from build123d import *

# Parameters (mm, degrees)
SKETCH1_R           = 4.78
BOSS_EXTRUDE1_DEPTH = 2.78
SKETCH2_W           = 6
SKETCH2_H           = 6
BOSS_EXTRUDE2_DEPTH = 10


with BuildPart() as part:
    # Sketch1 → Boss-Extrude1 (new, symmetric)
    with BuildSketch(Plane(origin=(0, 0, 0), x_dir=(0, 0, -1), z_dir=(1, 0, 0))):
        Circle(SKETCH1_R)
    extrude(amount=BOSS_EXTRUDE1_DEPTH, both=True)

    # Sketch2 → Boss-Extrude2 (add)
    with BuildSketch(Plane(origin=(2.78, 0, 0), x_dir=(0, 0, -1), z_dir=(1, 0, 0))):
        Rectangle(SKETCH2_W, SKETCH2_H)
    extrude(amount=BOSS_EXTRUDE2_DEPTH)


solid = part.part
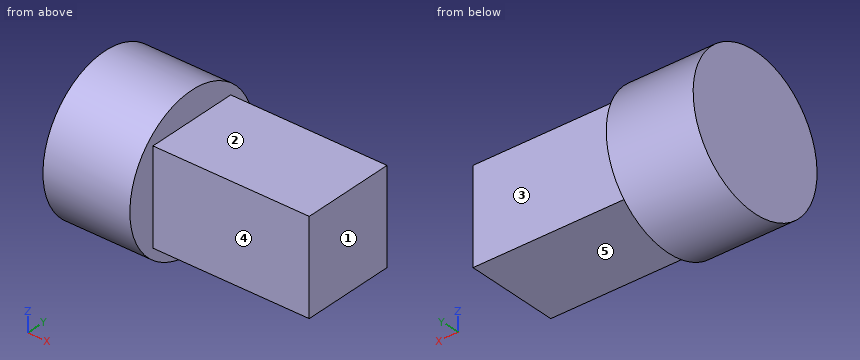
For this review, take the finished solid that the model builds, in its own axes (mm). Face numbers are marked on the shaded views. A direction names the side the tool comes from. Round coordinates to 2 decimals unless told otherwise and drop trailing zeros. Order: outer loops, then holes, each group sorted by start corner. A loop starts at its lowest first (then second) coordinate and runs counter-clockwise, first axis right, second up. Notation, with made-up numbers: (72.5, 14.25) -> (117.5, 14.25) arc R19 ccw to (117.5, 50.25) -> close; hole circle Ø2 at (74.25, 11.5). An arc over 180 degrees is marked (long way). Put each result on its own line as item: value.
Q1. Add section A-A on y = 0. Write out the cut boundary in (x, z).
Check result:
outline: (-2.78, -4.78) -> (2.78, -4.78) -> (2.78, -3) -> (12.78, -3) -> (12.78, 3) -> (2.78, 3) -> (2.78, 4.78) -> (-2.78, 4.78) -> close
Q2. Add section B-B on z = -1. Write out the cut boundary in (x, y).
Check result:
outline: (-2.78, -4.67) -> (2.78, -4.67) -> (2.78, -3) -> (12.78, -3) -> (12.78, 3) -> (2.78, 3) -> (2.78, 4.67) -> (-2.78, 4.67) -> close
Q3. Insertion check: pin 1 Ø5 at (x, z) = (10, 0.5) entering from -Y; pin 2 Ø3 at (x, y) = (6, -1) entering from +Z; pin 3 Ø3 at (x, y) = (10, 0) entering from -Z. Each pin has a flat end and moves straight along its axis. Give the tip position at first contact, or say it passes through.
Check result:
pin 1: y = -3
pin 2: z = 3
pin 3: z = -3
Q4. Add section C-C on x = 9. Write out the cut boundary in (y, z), plus the area to 3 significant figures.
Check result:
outline: (-3, -3) -> (3, -3) -> (3, 3) -> (-3, 3) -> close
area: 36.0 mm2
Q5. For probe 1 along Y at (x, z) = (12, 1.75); probe 2 along X at (y, z) = (-2.75, 3.25), list the stretches that pass through material, from the lowest coordinate up. Write a range as [from, to].
Check result:
probe 1: [-3, 3]
probe 2: [-2.78, 2.78]
Q6. Add section D-D on y = -3.75. Write out the cut boundary in (x, z).
Check result:
outline: (-2.78, -2.96) -> (2.78, -2.96) -> (2.78, 2.96) -> (-2.78, 2.96) -> close
Q7. Machinability: for the marked faces 1, 2, 3, 4 and 5, which of the approach directions +Z, -Z, +X, -X, +Y, -Y give a long, thin tool a straight path to every point of the face, cutting with its end or side? Answer none if there is none.
Check result:
face 1: +Z, -Z, +X, +Y, -Y
face 2: +Z, +X, +Y, -Y
face 3: +Z, -Z, +X, +Y
face 4: +Z, -Z, +X, -Y
face 5: -Z, +X, +Y, -Y
